Source: three-view drawing plus pictorial views. Frame: mm from the lowest corner of the part. Round coordinates to 2 decimals unless told otherwise and drop trailing zeros. Write each loop counter-clockwise with the first axis right and the second up, starting at its lowest first coordinate (ties: lowest second). Pieces come first, ordered by that corner, then holes. Notation, with made-up numbers: M -30,20 L -4,20 A8 cw -4,28 Z; hole C 20,4 d9. An arc over 180 degrees is marked long. Put each result on its own line as item: value. Start each with the question number.
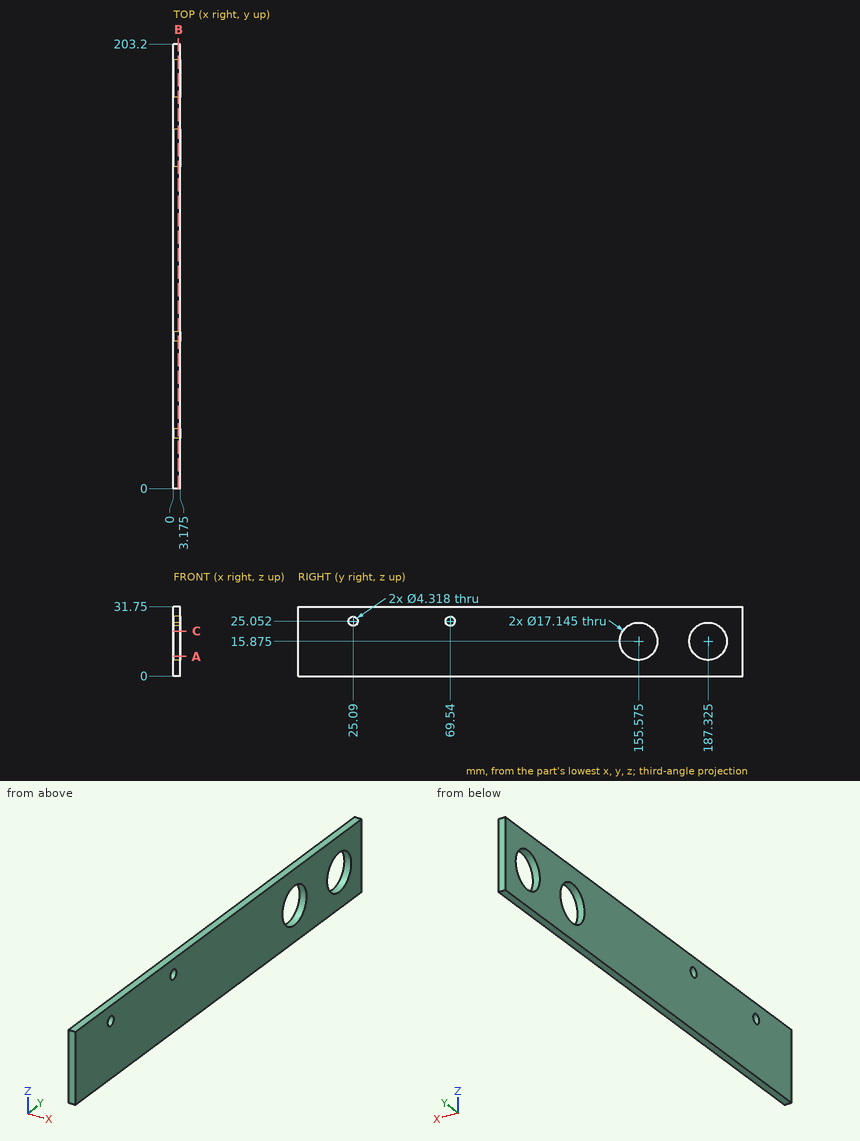
(1) Contact query for a flat-ended pin moving along its axis: P1, Ø3.5, axis at y = 69.54, z = 25.05, coming from the -X side. Output: stop coordinate, or through.
(2) Section query C-C (z = 20.5). Return loops of the section in (x, y) (3 decimals).
(3) Section query B-B (x = 2.3). Count the separate pieces of the cut face and the enclosed holes in it, and give its area (3 significant figures).
(4) Section query A-A (z = 9). Return loops of the section in (x, y) (3 decimals).
(5) Ray query, line 1 along Y through (x, z) = (0.7, 16); line 2 along Y through (x, z) = (0.9, 11); line 3 along Z through (x, y) = (2.25, 190). Return the intervals inside material, ascending.
Entries:
1. P1: through
2. outline: M 0,0 L 3.175,0 L 3.175,148.357 L 0,148.357 Z; M 0,162.793 L 3.175,162.793 L 3.175,180.107 L 0,180.107 Z; M 0,194.543 L 3.175,194.543 L 3.175,203.2 L 0,203.2 Z
3. separate pieces: 1
3. enclosed holes: 4
3. area: 5,960 mm2
4. outline: M 0,0 L 3.175,0 L 3.175,150.454 L 0,150.454 Z; M 0,160.696 L 3.175,160.696 L 3.175,182.204 L 0,182.204 Z; M 0,192.446 L 3.175,192.446 L 3.175,203.2 L 0,203.2 Z
5. line 1: 0 to 147, 164.15 to 178.75, 195.9 to 203.2
5. line 2: 0 to 148.52, 162.63 to 180.27, 194.38 to 203.2
5. line 3: 0 to 7.73, 24.02 to 31.75
